from build123d import *

# Parameters (mm, degrees)
ESBO_O1_W                = 56
ESBO_O1_H                = 37
RESSALTO_EXTRUS_O1_DEPTH = 3
ESBO_O10_W               = 3
ESBO_O10_H               = 37
RESSALTO_EXTRUS_O2_DEPTH = 13
ESBO_O13_W               = 3
ESBO_O13_H               = 37
RESSALTO_EXTRUS_O3_DEPTH = 13
ESBO_O14_R               = 5.84268935
CORTE_EXTRUS_O1_DEPTH    = 30
ESBO_O15_R               = 1.4
CORTE_EXTRUS_O2_DEPTH    = 60
ESBO_O17_R               = 1.4
CORTE_EXTRUS_O3_DEPTH    = 60


with BuildPart() as part:
    # Esboço1 → Ressalto-extrusão1 (new body)
    with BuildSketch(Plane(origin=(0, 0, 0), x_dir=(1, 0, 0), z_dir=(0, 1, 0))):
        with Locations((18.614655485, 40.673930531)):
            Rectangle(ESBO_O1_W, ESBO_O1_H)
    extrude(amount=RESSALTO_EXTRUS_O1_DEPTH)

    # Esboço10 → Ressalto-extrusão2 (add)
    with BuildSketch(Plane(origin=(0, 3, 0), x_dir=(1, 0, 0), z_dir=(0, 1, 0))):
        with Locations((-7.885344515, 40.673930531)):
            Rectangle(ESBO_O10_W, ESBO_O10_H)
    extrude(amount=RESSALTO_EXTRUS_O2_DEPTH)

    # Esboço13 → Ressalto-extrusão3 (add)
    with BuildSketch(Plane(origin=(0, 3, 0), x_dir=(1, 0, 0), z_dir=(0, 1, 0))):
        with Locations((45.114655485, 40.673930531)):
            Rectangle(ESBO_O13_W, ESBO_O13_H)
    extrude(amount=RESSALTO_EXTRUS_O3_DEPTH)

    # Esboço14 → Corte-extrusão1 (cut)
    with BuildSketch(Plane.ZY.offset(9.385344515)):
        with Locations((-41.314070298, 17.859240249)):
            Circle(ESBO_O14_R)
    extrude(amount=-CORTE_EXTRUS_O1_DEPTH, mode=Mode.SUBTRACT)

    # Esboço15 → Corte-extrusão2 (cut)
    with BuildSketch(Plane.ZY.offset(9.385344515)):
        with Locations((-27.173930531, 8)):
            Circle(ESBO_O15_R)
    extrude(amount=-CORTE_EXTRUS_O2_DEPTH, mode=Mode.SUBTRACT)

    # Esboço17 → Corte-extrusão3 (cut)
    with BuildSketch(Plane.ZY.offset(9.385344515)):
        with Locations((-54.173930531, 8)):
            Circle(ESBO_O17_R)
    extrude(amount=-CORTE_EXTRUS_O3_DEPTH, mode=Mode.SUBTRACT)


solid = part.part
Model file for the job. Use its own axes, mm. A direction names the side the tool comes from. Give positions to 0.01 mm unless a question says otherwise; leave off trailing zeros. Loops run counter-clockwise (first coordinate to the right, second up) from the corner with the lowest first, then second, coordinate; pieces in that order, holes last. Notation, with made-up numbers: (86.5, -36.5) -> (132.5, -36.5) arc R21 cw to (132.5, -12.5) -> close; hole circle Ø10 at (-33.75, -28). An arc over 180 degrees is marked (long way). Use a Markdown table: item, result. Add a question column.
(1) Drop flat-ended pins along their axis: pin 1 Ø2 at (y, z) = (8, -54.17) entering from -X; pin 2 Ø8 at (x, z) = (11.5, -55.5) entering from +Y. Give the stop position or say it passes through.
(2) Tool access for faces 1 (the cylindrical face through (-7.906, 7.148, -28.285)), 2 (the flat face through (18, 3, -41)), 3 (the cylindrical face through (-7.906, 12.017, -41.416)): list every direction of +Z, -Z, +X, -X, +Y, -Y with a clear straight run to the whole face (end or side of a thin tool).
(3) Slice it at C-C on x = 14. List the corners of the cut face in (y, z).
(4) Wall check: line 1 along X through (y, z) = (5.75, -31); line 2 along Y through (x, z) = (28.5, -24.5). Give the ranges that are in metal, low to high.
(5) Slice it at A-A on y = 10. List the corners of the cut face in (x, z), and give its area (3 significant figures).
(6) Mould opens along X. For faces 4 (the flat face through (43.615, 9, -40)), 5 (the flat face through (46.615, 8, -40)), 6 (the flat face through (16, 2, -22.174)), 7 (the flat face through (-9.385, 8, -40)) say: +X half, -X half, draft (parallel to the pull), parting line (faces both ways), or undercut.
(7) Slice it at B-B on z = -33. List the corners of the cut face in (x, y), and give its area (3 significant figures).
(8) Slice it at D-D on z = -44. List the corners of the cut face in (x, y), and give its area (3 significant figures).
Filled sheet:
| question | item | result |
|---|---|---|
| 1 | pin 1 | through |
| 1 | pin 2 | y = 3 |
| 2 | face 1 | +X, -X |
| 2 | face 2 | +Z, -Z, +Y |
| 2 | face 3 | -X, +Y |
| 3 | outline | (0, -59.17) -> (3, -59.17) -> (3, -22.17) -> (0, -22.17) -> close |
| 4 | line 1 | -9.39 to -6.39, 43.61 to 46.61 |
| 4 | line 2 | 0 to 3 |
| 5 | outline | (-9.39, -59.17) -> (-6.39, -59.17) -> (-6.39, -22.17) -> (-9.39, -22.17) -> close; (43.61, -59.17) -> (46.61, -59.17) -> (46.61, -22.17) -> (43.61, -22.17) -> close |
| 5 | area | 222 mm2 |
| 6 | face 4 | undercut |
| 6 | face 5 | +X half |
| 6 | face 6 | draft |
| 6 | face 7 | -X half |
| 7 | outline | (-9.39, 0) -> (46.61, 0) -> (46.61, 16) -> (43.61, 16) -> (43.61, 3) -> (-6.39, 3) -> (-6.39, 16) -> (-9.39, 16) -> close |
| 7 | area | 246 mm2 |
| 8 | outline | (-9.39, 0) -> (46.61, 0) -> (46.61, 16) -> (43.61, 16) -> (43.61, 3) -> (-6.39, 3) -> (-6.39, 12.67) -> (-9.39, 12.67) -> close |
| 8 | area | 236 mm2 |
